Read the model definition and answer for the solid it produces. Units are mm, in the model's axes. A direction names the side the tool comes from. Round coordinates to 2 decimals unless told otherwise and drop trailing zeros. Write each loop counter-clockwise with the first axis right and the second up, starting at its lowest first coordinate (ties: lowest second). Pieces come first, ordered by that corner, then holes. Notation, with made-up numbers: (58.25, 10) -> (70.25, 10) arc R20 cw to (70.25, 37) -> close; hole circle Ø2 at (41, 88.25). An arc over 180 degrees is marked (long way). Return JSON: item names as keys, results as strings. Group by question number.
(1) The mould has two halves that part along X. Classify faces 1 (the flat face through (10, 10, 2)), 2 (the flat face through (15, 16.5, 6.6)), 3 (the flat face through (2, 20, 6)), 4 (the flat face through (0, 30, 3)): released by +X, released by -X, zero draft, split by the parting line, or undercut.
(2) For faces 5 (the cylindrical face through (17.54, 14.47, 5.38)), 6 (the flat face through (17, 20, 6)), 7 (the cylindrical face through (11.48, 12.32, 3.48)), 8 (the flat face through (9, 7, 5)), 9 (the cylindrical face through (2.54, 14.47, 5.38)), determine the directions among +Z, -Z, +X, -X, +Y, -Y from which every point of the face is accessible in a straight line to the end or side of a thin tool.
(3) A cutting plane is placed at B-B on z = 5.75. Give the vertices of the cut face in (x, y).
(4) A cutting plane is placed at C-C on x = 10. Give the vertices of the cut face in (y, z).
(5) Given pin 1 (9 mm diameter, centred on x = 10.5, y = 11, fed in from +Z); pin 2 (1.3 mm diameter, centred on x = 18, z = 7, fed in from +Y); pin 3 (0.6 mm diameter, centred on x = 3.5, z = 7, fed in from -Y), each flat-ended and moving along its own axis, determine where each tip first touches the part or whether it passes through.
(6) A cutting plane is placed at A-A on y = 40. Give the vertices of the cut face in (x, z), then the cut area to 3 significant figures.
(7) A cutting plane is placed at D-D on y = 12. Give the vertices of the cut face in (x, z).
(8) Straight lines are drawn through the part: line 1 (X direction, y = 40, z = 3.5); line 2 (Z direction, x = 1.8, y = 17.5); line 3 (X direction, y = 15.5, z = 6.25). For each, find the intervals that lie inside material, in ascending order.
```python
from build123d import *

# Parameters (mm, degrees)
F0_W         = 20
F0_H         = 60
F0_R         = 4
F0_R_2       = 6.05
F1_DEPTH     = 4
F1_FACE_W    = 20
F1_FACE_H    = 60
F1_FACE_R    = 4
F1_FACE_R_2  = 6.05
F0_R_3       = 2.75
F2_DEPTH     = 1
F3_W         = 5
F3_H         = 5
F4_DEPTH     = 5
F5_T1_DEPTH  = 97.9025398997
F6_R         = 2.49999
F7_R         = 1.1
F8_DEPTH     = 25
F9_DEPTH     = 5
F10_T1_DEPTH = 97.8518303197
F11_DEPTH    = 2


# Not quite as in the source:
# - a fillet or chamfer that OpenCascade refuses, or shapes differently, is made with other operations: its cross-section is extruded or revolved along the edge and cut away or added
# - a fillet or chamfer is up to 0.001 mm smaller than in the source, because OpenCascade refuses the exact size


with BuildPart() as f1:
    # F0 (on Top) → F1 (new body)
    with BuildSketch(Plane.XY):
        with Locations((10, 30)):
            Rectangle(F0_W, F0_H)
        with Locations((10, 10)):
            Circle(F0_R, mode=Mode.SUBTRACT)
        with Locations((10, 40)):
            Circle(F0_R_2, mode=Mode.SUBTRACT)
    extrude(amount=F1_DEPTH)

    # F1_face (on face) + F0 (on Top) → F2 (join)
    with BuildSketch(Plane(origin=(10, 29.8602632633, 4), x_dir=(1, 0, 0), z_dir=(0, 0, 1))):
        with Locations((0, 0.1397367367)):
            Rectangle(F1_FACE_W, F1_FACE_H)
        with Locations((0, -19.8602632633)):
            Circle(F1_FACE_R, mode=Mode.SUBTRACT)
        with Locations((0, 10.1397367367)):
            Circle(F1_FACE_R_2, mode=Mode.SUBTRACT)
    with BuildSketch(Plane.XY):
        with Locations((10, 10)):
            Circle(F0_R)
        with Locations((10, 10)):
            Circle(F0_R_3, mode=Mode.SUBTRACT)
    extrude(amount=F2_DEPTH)

    # F3 (on face) → F4 (join)
    with BuildSketch(Plane.XY.offset(5)):
        with Locations((2.5, 17.5)):
            Rectangle(F3_W, F3_H)
        with Locations((17.5, 17.5)):
            Rectangle(F3_W, F3_H)
    extrude(amount=F4_DEPTH)

    # F5: chamfer of 15 x 4 on 1 edges, made by hand

    # F5_s2 → F5_t1 (cut)
    with BuildSketch(Plane.YZ.offset(-38.9512699498)):
        Polygon((15, 5), (0, 1), (0, 5), align=None)
    extrude(amount=F5_T1_DEPTH, mode=Mode.SUBTRACT)

    # F6 (radius 2.5 in the source; OpenCascade refuses exactly that, so slightly less here)
    f6_edges = [f1.edges().sort_by_distance(p)[0] for p in [
        (2.5, 15, 5),
        (2.5, 15, 10),
        (17.5, 15, 5),
        (17.5, 15, 10),
        (2.5, 20, 10),
        (17.5, 20, 10),
    ]]
    fillet(f6_edges, radius=F6_R)

    # F7 (on face) → F8 (cut)
    with BuildSketch(Plane(origin=(0, 0, 0), x_dir=(0, -1, 0), z_dir=(-1, 0, 0))):
        with Locations((-17.5, 7.5)):
            Circle(F7_R)
    extrude(amount=-F8_DEPTH, mode=Mode.SUBTRACT)

    # F10: chamfer of 5 x 15 on 1 edges, made by hand

    # F10_s2 → F10_t1 (cut)
    with BuildSketch(Plane.YZ.offset(-38.9259151598)):
        Polygon((60, 0), (45, 5), (60, 5), align=None)
    extrude(amount=F10_T1_DEPTH, mode=Mode.SUBTRACT)



with BuildPart() as f9:
    # F0 (on Top) → F9 (new body)
    with BuildSketch(Plane.XY):
        with Locations((10, 10)):
            Circle(F0_R)
        with Locations((10, 10)):
            Circle(F0_R_3, mode=Mode.SUBTRACT)
    extrude(amount=F9_DEPTH)


with BuildPart() as f1_1:
    add(f1.part)

    add(f9.part)  # F11 merges F9
    # F0 (on Top) → F11 (join)
    with BuildSketch(Plane.XY):
        with Locations((10, 10)):
            Circle(F0_R_3)
    extrude(amount=F11_DEPTH)


solid = f1_1.part
```
Checks:
{
 "1": {"face 1": "undercut", "face 2": "undercut", "face 3": "zero draft", "face 4": "released by -X"},
 "2": {"face 5": "+Z, +X, -Y", "face 6": "+Z, +X, -X, +Y", "face 7": "+Z", "face 8": "+Z, +X, -X, +Y, -Y", "face 9": "+Z, -X, -Y"},
 "3": {"outline": "(0, 14.71) -> (5, 14.71) -> (5, 20) -> (0, 20) -> close; (15, 14.71) -> (20, 14.71) -> (20, 20) -> (15, 20) -> close"},
 "4": {"outline": "(0, 0) -> (33.95, 0) -> (33.95, 5) -> (15, 5) -> (14, 4.73) -> (14, 5) -> (12.75, 5) -> (12.75, 2) -> (7.25, 2) -> (7.25, 5) -> (6, 5) -> (6, 2.6) -> (0, 1) -> close; (46.05, 0) -> (60, 0) -> (46.05, 4.65) -> close"},
 "5": {"pin 1": "stops at z = 5", "pin 2": "stops at y = 20", "pin 3": "stops at y = 14.99"},
 "6": {"outline": "(0, 0) -> (3.95, 0) -> (3.95, 5) -> (0, 5) -> close; (16.05, 0) -> (20, 0) -> (20, 5) -> (16.05, 5) -> close", "area": "39.5 mm^2"},
 "7": {"outline": "(0, 0) -> (20, 0) -> (20, 4.2) -> (13.46, 4.2) -> (13.46, 5) -> (11.89, 5) -> (11.89, 2) -> (8.11, 2) -> (8.11, 5) -> (6.54, 5) -> (6.54, 4.2) -> (0, 4.2) -> close"},
 "8": {"line 1": "x = 0 to 3.95, 16.05 to 20", "line 2": "z = 0 to 6.4, 8.6 to 10", "line 3": "x = 0 to 5, 15 to 20"}
}
